from build123d import *

# Parameters (mm, degrees)
CROQUIS2_R = 9.75


with BuildPart() as part:
    # Barrer1: sweep along a path in Croquis1
    with BuildLine(Plane.XY) as barrer1_path:
        Line((0, 0), (0, 150))
        ThreePointArc((0, 150), (29.289321881, 220.710678119), (100, 250))
        Line((100, 250), (249, 250))
        ThreePointArc((249, 250), (319.710678119, 220.710678119), (349, 150))
        Line((349, 150), (349, 0))
    # Croquis2 → Barrer1 (sweep)
    with BuildSketch(Plane(origin=(0, 0, 0), x_dir=(1, 0, 0), z_dir=(0, 1, 0))):
        Circle(CROQUIS2_R)
    sweep(path=barrer1_path.line)


solid = part.part
Design review of the part built by this model. Coordinates are the model's own, in mm. A direction names the side the tool comes from. Give positions to 0.01 mm unless a question says otherwise; leave off trailing zeros. Order: outer loops, then holes, each group sorted by start corner. A loop starts at its lowest first (then second) coordinate and runs counter-clockwise, first axis right, second up. Notation, with made-up numbers: (5, -22.5) - (25, -22.5) arc R26 ccw to (25, -6.5) - close; hole circle Ø2 at (68.5, 38). An arc over 180 degrees is marked (long way). Use CSV: the item, a comma, the result in double quotes. Start each with the question number.
Q1. Machinability: for faces 3 (the face through (175.54, 259.74, -0.43)), 4 (the face through (349, 0, 0)), 5 (the face through (-1.269, 76.05, -9.667)), which of the approach directions +Z, -Z, +X, -X, +Y, -Y give a long, thin tool a straight path to every point of the face, cutting with its end or side? Answer none if there is none.
Q2. Draft analysis for pull direction X (two halves, no side actions). For faces 1 (the face through (339.7, 73.95, -2.93)), 2 (the face through (0, 0, 0)), state which applies: pulls with the +X half, pulls with the -X half, needs draft (parallel to the pull), parting line crosses it, or undercut.
Q3. Take a section at C-C (x = 236). State the section outline as (y, z) points.
Q4. For P1, Ø6, axis at x = 316.5, z = 6.5, coming from the -Y side; P2, Ø4, axis at x = 200.5, z = -6.5, coming from the -Y side; P3, Ø2, axis at x = 230.5, z = 4.5, coming from the +Y side, all flat-tipped, find the tip position at first contact; note any pin that passes through.
Q5. For line 1 (X direction, y = 108, z = -1); line 2 (X direction, y = 177.5, z = -4.5); line 3 (Y direction, x = 122, z = -0.25), list the stretches that pass through material, from the lowest coordinate up.
Q6. Take a section at A-A (y = 107). State the section outline as (x, z) points.
Q7. Take a section at B-B (z = 0). State the section outline as (x, y) points, and give its area (3 significant figures).
Calculated:
1,face 3,"none"
1,face 4,"+Z, -Z, +X, -X, -Y"
1,face 5,"-Y"
2,face 1,"undercut"
2,face 2,"needs draft"
3,outline,"circle Ø19.5 at (250, 0)"
4,P1,"stops at y = 208.98"
4,P2,"stops at y = 241.35"
4,P3,"stops at y = 259.1"
5,line 1,"x = -9.7 to 9.7, 339.3 to 358.7"
5,line 2,"x = -5.11 to 12.89, 336.11 to 354.11"
5,line 3,"y = 240.25 to 259.75"
6,outline,"circle Ø19.5 at (0, 0); circle Ø19.5 at (349, 0)"
7,outline,"(-9.75, 0) - (9.75, 0) - (9.75, 150) arc R90.25 cw to (100, 240.25) - (249, 240.25) arc R90.25 cw to (339.25, 150) - (339.25, 0) - (358.75, 0) - (358.75, 150) arc R109.75 ccw to (249, 259.75) - (100, 259.75) arc R109.75 ccw to (-9.75, 150) - close"
7,area,"14,900 mm²"
